For this review, take the finished solid that the model builds, in its own axes (mm). Face numbers are marked on the shaded views. A direction names the side the tool comes from. Coordinates: 2 decimals unless noted, no trailing zeros. Order: outer loops, then holes, each group sorted by start corner. A loop starts at its lowest first (then second) coordinate and runs counter-clockwise, first axis right, second up.
from build123d import *

# Parameters (mm, degrees)
SKETCH_1_R          = 2
SKETCH_1_R_2        = 1
EXTRUDE_1_DEPTH     = 29
SKETCH_2_R          = 3
SKETCH_2_R_2        = 2
EXTRUDE_2_DEPTH     = 2.5
EXTRUDE_START       = 26.5
SKETCH_3_R          = 3
SKETCH_3_R_2        = 2
EXTRUDE_3_DEPTH     = 2.5
SKETCH_4_R          = 1.6
CUT_EXTRUDE_1_DEPTH = 1.5
CUT_EXTRUDE_START   = 29
CUT_EXTRUDE_2_DEPTH = 1.6
SKETCH_7_R          = 3
CUT_EXTRUDE_3_DEPTH = 10.5
CUT_EXTRUDE_START_2 = 10.5
CUT_EXTRUDE_4_DEPTH = 8


with BuildPart() as part:
    # 草图1 → 凸台-拉伸1 (new body)
    with BuildSketch(Plane(origin=(0, 0, 0), x_dir=(1, 0, 0), z_dir=(0, 1, 0))):
        with Locations(Location((0, 0, 0), (0, 0, 90))):
            Circle(SKETCH_1_R)
        with Locations(Location((0, 0, 0), (0, 0, 90))):
            Circle(SKETCH_1_R_2, mode=Mode.SUBTRACT)
    extrude(amount=EXTRUDE_1_DEPTH)

    # 草图2 → 凸台-拉伸2 (add)
    with BuildSketch(Plane(origin=(0, 0, 0), x_dir=(1, 0, 0), z_dir=(0, 1, 0))):
        with Locations(Location((0, 0, 0), (0, 0, 270))):
            Circle(SKETCH_2_R)
        with Locations(Location((0, 0, 0), (0, 0, 90))):
            Circle(SKETCH_2_R_2, mode=Mode.SUBTRACT)
    extrude(amount=EXTRUDE_2_DEPTH)

    # 草图3 → 凸台-拉伸3 (add)
    with BuildSketch(Plane(origin=(0, 0, 0), x_dir=(1, 0, 0), z_dir=(0, 1, 0)).offset(EXTRUDE_START)):
        with Locations(Location((0, 0, 0), (0, 0, 270))):
            Circle(SKETCH_3_R)
        with Locations(Location((0, 0, 0), (0, 0, 90))):
            Circle(SKETCH_3_R_2, mode=Mode.SUBTRACT)
    extrude(amount=EXTRUDE_3_DEPTH)

    # 草图4 → 切除-拉伸1 (cut)
    with BuildSketch(Plane(origin=(0, 0, 0), x_dir=(1, 0, 0), z_dir=(0, 1, 0))):
        with Locations(Location((0, 0, 0), (0, 0, 270))):
            Circle(SKETCH_4_R)
    extrude(amount=CUT_EXTRUDE_1_DEPTH, mode=Mode.SUBTRACT)

    # 草图5 → 切除-拉伸2 (cut)
    with BuildSketch(Plane(origin=(0, 0, 0), x_dir=(1, 0, 0), z_dir=(0, 1, 0)).offset(CUT_EXTRUDE_START)):
        Polygon((0, -2.309401077), (2, -1.154700538), (2, 1.154700538), (0, 2.309401077), (-2, 1.154700538), (-2, -1.154700538), align=None)
    extrude(amount=-CUT_EXTRUDE_2_DEPTH, mode=Mode.SUBTRACT)

    # 草图7 → 切除-拉伸3 (cut)
    with BuildSketch(Plane(origin=(0, 0, 0), x_dir=(1, 0, 0), z_dir=(0, 1, 0))):
        with Locations(Location((0, 0, 0), (0, 0, 270))):
            Circle(SKETCH_7_R)
    extrude(amount=CUT_EXTRUDE_3_DEPTH, mode=Mode.SUBTRACT)

    # 草图8 → 切除-拉伸4 (cut)
    with BuildSketch(Plane(origin=(0, 0, 0), x_dir=(1, 0, 0), z_dir=(0, 1, 0)).offset(CUT_EXTRUDE_START_2)):
        with BuildLine():
            Line((0, 0), (2, 0))
            ThreePointArc((2, 0), (1.414213562, 1.414213562), (0, 2))
            Line((0, 2), (0, 0))
        make_face()
        with BuildLine():
            Line((0, -2), (0, 0))
            Line((0, 0), (-2, 0))
            ThreePointArc((-2, 0), (-1.414213562, -1.414213562), (0, -2))
        make_face()
    extrude(amount=CUT_EXTRUDE_4_DEPTH, mode=Mode.SUBTRACT)


solid = part.part
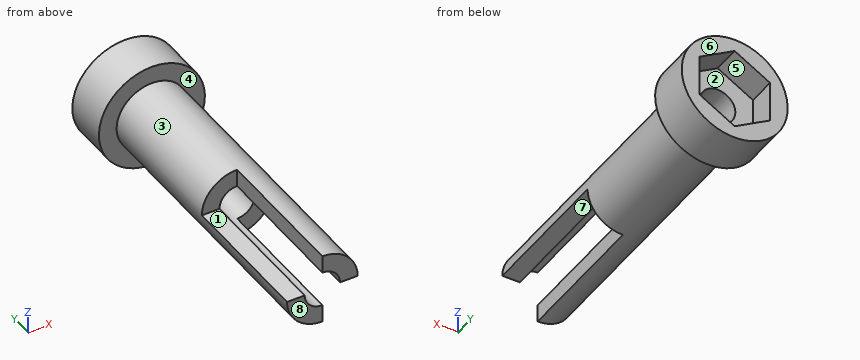
1. Machinability: for the marked faces 4, 5, 6, 7 and 8, which of the approach directions +Z, -Z, +X, -X, +Y, -Y give a long, thin tool a straight path to every point of the face, cutting with its end or side? Answer none if there is none.
Answer below:
face 4: -Y
face 5: +Y
face 6: +Z, -Z, +X, -X, +Y
face 7: -Z, +X, -Y
face 8: +Z, -Z, +X, -X, -Y
2. Clearance check with flat-ended pins moving along their axes: pin 1 Ø1 at (x, y) = (-1, 20) entering from -Z; pin 2 Ø0.5 at (y, z) = (14.5, -1.5) entering from +X; pin 3 Ø2 at (y, z) = (13, 1.5) entering from -X. State where each tip first meets the part, or that it passes through.
Answer below:
pin 1: stops at z = -1.94
pin 2: stops at x = 0
pin 3: stops at x = 0
3. Take a section at D-D, the plane y = 26. Give the boundary of the cut face in (x, z), plus the area to 3 significant figures.
Answer below:
outline: circle Ø4 at (0, 0); hole circle Ø2 at (0, 0)
area: 9.42 mm2
4. Take a section at C-C, the plane x = -1.5. Give the boundary of the cut face in (y, z), plus the area to 3 significant figures.
Answer below:
outline: (10.5, -1.32) - (26.5, -1.32) - (26.5, -2.6) - (29, -2.6) - (29, -1.44) - (27.4, -1.44) - (27.4, 1.44) - (29, 1.44) - (29, 2.6) - (26.5, 2.6) - (26.5, 1.32) - (18.5, 1.32) - (18.5, 0) - (10.5, 0) - close
area: 40.1 mm2
5. The part is to be moulded in two halves that separate along X. For the marked faces 1, 2 and 3, say which applies: +X half, -X half, draft (parallel to the pull), parting line (faces both ways), or undercut.
Answer below:
face 1: draft
face 2: undercut
face 3: parting line
6. Take a section at A-A, the plane y = 17.75. Give the boundary of the cut face in (x, z).
Answer below:
outline: (-2, 0) arc R2 ccw to (0, -2) - (0, -1) arc R1 cw to (-1, 0) - close; (0, 1) arc R1 cw to (1, 0) - (2, 0) arc R2 ccw to (0, 2) - close
7. Take a section at B-B, the plane z = -0.3. Give the boundary of the cut face in (x, y).
Answer below:
outline: (-2.98, 26.5) - (-1.98, 26.5) - (-1.98, 10.5) - (-0.95, 10.5) - (-0.95, 27.4) - (-2, 27.4) - (-2, 29) - (-2.98, 29) - close; (0.95, 18.5) - (1.98, 18.5) - (1.98, 26.5) - (2.98, 26.5) - (2.98, 29) - (2, 29) - (2, 27.4) - (0.95, 27.4) - close
8. To check wall thickness, follow L1, parallel to X at y = 18, z = -0.1; L2, parallel to X at y = 19, z = 0; L3, parallel to Y at x = 2.35, z = 0.15. State the ranges of each line that lie inside material, in increasing order.
Answer below:
L1: x = -2 to -0.99
L2: x = -2 to -1, 1 to 2
L3: y = 26.5 to 29
